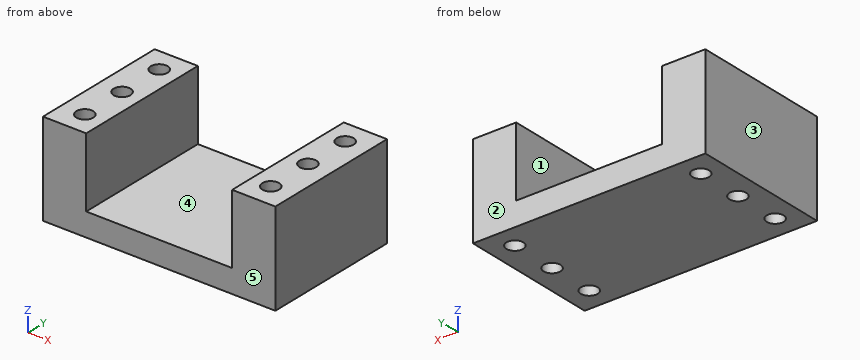
```python
from build123d import *

# Parameters (mm, degrees)
F0_W     = 11.811
F0_H     = 38.1
F0_R     = 2.3114
F1_DEPTH = 25.4
F0_W_2   = 39.878
F2_DEPTH = 6.35


with BuildPart() as f1:
    # F0 (on Top) → F1 (new body)
    with BuildSketch(Plane.XY):
        with Locations((-21.633447, 7.007305)):
            Rectangle(F0_W, F0_H)
        with Locations((-21.188947, -5.692695)):
            Circle(F0_R, mode=Mode.SUBTRACT)
        with Locations((-21.188947, 7.007305)):
            Circle(F0_R, mode=Mode.SUBTRACT)
        with Locations((-21.188947, 19.707305)):
            Circle(F0_R, mode=Mode.SUBTRACT)
        with Locations((30.055553, 7.007305)):
            Rectangle(F0_W, F0_H)
        with Locations((29.611053, -5.692695)):
            Circle(F0_R, mode=Mode.SUBTRACT)
        with Locations((29.611053, 7.007305)):
            Circle(F0_R, mode=Mode.SUBTRACT)
        with Locations((29.611053, 19.707305)):
            Circle(F0_R, mode=Mode.SUBTRACT)
    extrude(amount=F1_DEPTH)

    # F0 (on Top) → F2 (join)
    with BuildSketch(Plane.XY):
        with Locations((4.211053, 7.007305)):
            Rectangle(F0_W_2, F0_H)
    extrude(amount=F2_DEPTH)


solid = f1.part
```
Geometry check sheet. Reference: the model listing, model coordinates, mm. Face numbers are marked on the shaded views. A direction names the side the tool comes from. Round coordinates to 2 decimals unless told otherwise and drop trailing zeros. Loops run counter-clockwise (first coordinate to the right, second up) from the corner with the lowest first, then second, coordinate; pieces in that order, holes last. Notation, with made-up numbers: M -37,62 L -1,62 A36 cw -1,99 Z; hole C -29.5,85.25 d6. An arc over 180 degrees is marked long. Return JSON: item names as keys, results as strings. Group by question number.
(1) Mould release check, pull along X, two halves, no side actions. Record for the marked faces 3, 4 and 5: pulls with the +X half, pulls with the -X half, needs draft (parallel to the pull), parting line crosses it, or undercut.
(2) Scan lines: line 1 along X through (y, z) = (2, 19.25); line 2 along Y through (x, z) = (28, 21.5); line 3 along Y through (x, z) = (-22, 22.25). Record each from-to range of solid material in increasing order. Write a range as [from, to].
(3) Section check C-C, the plane y = -7. Enter the section's corners in (x, z).
(4) Section check D-D, the plane y = 4. Enter the section's corners in (x, z).
(5) Section check A-A, the plane z = 21.5. Enter the section's corners in (x, y).
(6) Section check B-B, the plane x = 30. Enter the section's corners in (y, z).
(7) Set-up check for the marked faces 1 and 2: record each of +Z, -Z, +X, -X, +Y, -Y from which the full face is reachable in a straight line by a thin tool's end or side.
(8) Go/stop test with flat-tipped pins: pin 1 (7.5 mm diameter, centred on x = 29.61, y = 19.71, fed in from +Z); pin 2 (10 mm diameter, centred on x = 6.5, y = 7.5, fed in from +Z). Record where each tip stops, or that it passes through.
Data:
{
 "1": {"face 3": "pulls with the -X half", "face 4": "undercut", "face 5": "needs draft"},
 "2": {"line 1": "[-27.54, -15.73], [24.15, 35.96]", "line 2": "[-12.04, -7.35], [-4.04, 5.35], [8.66, 18.05], [21.36, 26.06]", "line 3": "[-12.04, -7.86], [-3.53, 4.84], [9.17, 17.54], [21.87, 26.06]"},
 "3": {"outline": "M -27.54,0 L -23.1,0 L -23.1,25.4 L -27.54,25.4 Z; M -19.28,0 L 27.7,0 L 27.7,25.4 L 24.15,25.4 L 24.15,6.35 L -15.73,6.35 L -15.73,25.4 L -19.28,25.4 Z; M 31.52,0 L 35.96,0 L 35.96,25.4 L 31.52,25.4 Z"},
 "4": {"outline": "M -27.54,0 L 35.96,0 L 35.96,25.4 L 24.15,25.4 L 24.15,6.35 L -15.73,6.35 L -15.73,25.4 L -27.54,25.4 Z"},
 "5": {"outline": "M -27.54,-12.04 L -15.73,-12.04 L -15.73,26.06 L -27.54,26.06 Z; M 24.15,-12.04 L 35.96,-12.04 L 35.96,26.06 L 24.15,26.06 Z; hole C -21.19,-5.69 d4.62; hole C -21.19,7.01 d4.62; hole C -21.19,19.71 d4.62; hole C 29.61,-5.69 d4.62; hole C 29.61,7.01 d4.62; hole C 29.61,19.71 d4.62"},
 "6": {"outline": "M -12.04,0 L -7.97,0 L -7.97,25.4 L -12.04,25.4 Z; M -3.41,0 L 4.73,0 L 4.73,25.4 L -3.41,25.4 Z; M 9.29,0 L 17.43,0 L 17.43,25.4 L 9.29,25.4 Z; M 21.99,0 L 26.06,0 L 26.06,25.4 L 21.99,25.4 Z"},
 "7": {"face 1": "+Z, +Y, -Y", "face 2": "+Z, -Z, +X, -X, +Y"},
 "8": {"pin 1": "z = 25.4", "pin 2": "z = 6.35"}
}
